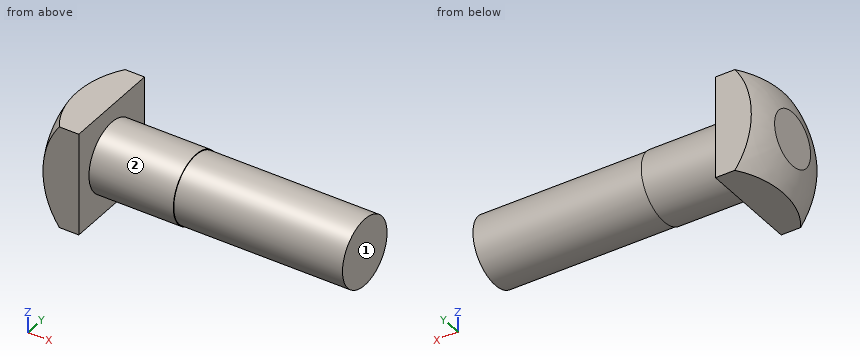
from build123d import *

# Parameters (mm, degrees)
SKETCH2_W      = 38.6744488
SKETCH2_H      = 37.46857502
EXTRUDE1_DEPTH = 16.6624


with BuildPart() as part:
    # Sketch1 → Revolve1 (revolve)
    with BuildSketch(Plane.XY, mode=Mode.PRIVATE) as revolve1_sk:
        Polygon((111.9124, 0), (16.6624, 0), (16.6624, 12.954), (48.4124, 12.954), (48.4124, 12.7), (111.9124, 12.7), align=None)
    revolve(revolve1_sk.sketch.rotate(Axis((0, 0, 0), (1, 0, 0)), 180), axis=Axis((0, 0, 0), (1, 0, 0)))

    # Sketch2 → Extrude1 (add)
    with BuildSketch(Plane(origin=(0, 0, 0), x_dir=(0, 0, -1), z_dir=(1, 0, 0))):
        Rectangle(SKETCH2_W, SKETCH2_H)
    extrude(amount=EXTRUDE1_DEPTH)

    # Sketch3 → Cut-Revolve1 (revolve, cut)
    with BuildSketch(Plane.XY, mode=Mode.PRIVATE) as cut_revolve1_sk:
        with BuildLine():
            Line((0, 0), (0, 10.258215468))
            ThreePointArc((0, 10.258215468), (5.469928088, 22.402987857), (15.210208347, 31.488280924))
            Line((15.210208347, 31.488280924), (-5.301244899, 31.488280924))
            Line((-5.301244899, 31.488280924), (-5.301244899, 0))
            Line((-5.301244899, 0), (0, 0))
        make_face()
    revolve(cut_revolve1_sk.sketch.rotate(Axis((0, 0, 0), (-1, 0, 0)), 90), axis=Axis((0, 0, 0), (-1, 0, 0)), mode=Mode.SUBTRACT)


solid = part.part
Input: part model. Units: mm. Frame: model coordinates. Face numbers are marked on the shaded views. A direction names the side the tool comes from. Coordinates: 2 decimals unless noted, no trailing zeros. Loops run counter-clockwise (first coordinate to the right, second up) from the corner with the lowest first, then second, coordinate; pieces in that order, holes last. Notation, with made-up numbers: (59.25, -4) -> (65.25, -4) arc R33 cw to (65.25, 28) -> close; hole circle Ø1 at (-20, -33). An arc over 180 degrees is marked (long way). One line per item, written item: value.
(1) Set-up query: the marked faces 1 and 2. Return all of +Z, -Z, +X, -X, +Y, -Y with unobstructed straight access to the full face (end or side cutting, diameter ignored); none if empty.
Answer below:
face 1: +Z, -Z, +X, +Y, -Y
face 2: +X
(2) Pin query (flat end, axial travel): pin 1 Ø1.5 at (x, z) = (70.5, 11) entering from +Y; pin 2 Ø5 at (x, z) = (63, -14) entering from +Y; pin 3 Ø10 at (x, z) = (84.5, -5) entering from +Y. Return the tip coordinate at first contact, or that it passes through.
Answer below:
pin 1: stops at y = 7.5
pin 2: stops at y = 5.39
pin 3: stops at y = 12.7
(3) Cut plane A-A (x = 26). Output: boundary loops of the cut face in (y, z), then the cut area to 3 significant figures.
Answer below:
outline: circle Ø25.91 at (0, 0)
area: 527 mm2
(4) Ray query, line 1 along Z through (x, y) = (65, 7.5); line 2 along Z through (x, y) = (50.5, -9.5); line 3 along Y through (x, z) = (28.5, 4.5). Return the intervals inside material, ascending.
Answer below:
line 1: z = -10.25 to 10.25
line 2: z = -8.43 to 8.43
line 3: y = -12.15 to 12.15
